from build123d import *

# Parameters (mm, degrees)
SKETCH2_R           = 17.4
SKETCH2_R_2         = 4.45
BOSS_EXTRUDE1_DEPTH = 4


with BuildPart() as part:
    # Sketch2 → Boss-Extrude1 (new body)
    with BuildSketch(Plane.XY):
        Polygon((53.044712849, 33.544372616), (42.778880935, 33.544372616), (42.778880935, 29.544372616), (2.778880935, 29.544372616), (2.778880935, 33.544372616), (-57.221119065, 33.544372616), (-57.221119065, 29.544372616), (-97.221119065, 29.544372616), (-97.221119065, 33.544372616), (-157.221119065, 33.544372616), (-157.221119065, 29.544372616), (-197.221119065, 29.544372616), (-197.221119065, 33.544372616), (-207.486950979, 33.544372616), (-217.221119065, -17.455627384), (-217.221119065, -21.455627384), (-197.221119065, -21.455627384), (-197.221119065, -17.455627384), (-157.221119065, -17.455627384), (-157.221119065, -21.455627384), (-97.221119065, -21.455627384), (-97.221119065, -17.455627384), (-57.221119065, -17.455627384), (-57.221119065, -21.455627384), (2.778880935, -21.455627384), (2.778880935, -17.455627384), (42.778880935, -17.455627384), (42.778880935, -21.455627384), (62.778880935, -21.455627384), (62.778880935, -17.455627384), align=None)
        with Locations((-105.221119065, 4.044372616)):
            Circle(SKETCH2_R, mode=Mode.SUBTRACT)
        with Locations((-130.864831745, -8.505627384)):
            Circle(SKETCH2_R_2, mode=Mode.SUBTRACT)
        with Locations((-79.577406385, 16.594372616)):
            Circle(SKETCH2_R_2, mode=Mode.SUBTRACT)
        with Locations((-74.864831745, -8.505627384)):
            Circle(SKETCH2_R_2, mode=Mode.SUBTRACT)
        with Locations((-49.221119065, 4.044372616)):
            Circle(SKETCH2_R, mode=Mode.SUBTRACT)
        with Locations((-23.577406385, 16.594372616)):
            Circle(SKETCH2_R_2, mode=Mode.SUBTRACT)
        with BuildLine():
            Line((-16.476478057, 4.792165998), (-25.639690827, -7.001469778))
            ThreePointArc((-25.639690827, -7.001469778), (-26.073848783, -11.213946123), (-22.481034397, -13.455627384))
            Line((-22.481034397, -13.455627384), (9.665493618, -13.455627384))
            ThreePointArc((9.665493618, -13.455627384), (13.553631861, -10.39497876), (11.491657622, -5.896817888))
            Line((11.491657622, -5.896817888), (-11.491657622, 5.896817888))
            ThreePointArc((-11.491657622, 5.896817888), (-14.183239425, 6.243267926), (-16.476478057, 4.792165998))
        make_face(mode=Mode.SUBTRACT)
        with BuildLine():
            Line((-165.933895752, 18.177294134), (-142.950580507, 6.383658359))
            ThreePointArc((-142.950580507, 6.383658359), (-140.258998705, 6.03720832), (-137.965760073, 7.488310249))
            Line((-137.965760073, 7.488310249), (-128.802547302, 19.281946025))
            ThreePointArc((-128.802547302, 19.281946025), (-128.368389347, 23.49442237), (-131.961203733, 25.736103631))
            Line((-131.961203733, 25.736103631), (-164.107731748, 25.736103631))
            ThreePointArc((-164.107731748, 25.736103631), (-167.995869991, 22.675455007), (-165.933895752, 18.177294134))
        make_face(mode=Mode.SUBTRACT)
        with BuildLine():
            Line((38.778880935, -4.35874426), (38.778880935, 23.243985793))
            ThreePointArc((38.778880935, 23.243985793), (37.232462018, 26.403090076), (33.788911001, 27.119545047))
            Line((33.788911001, 27.119545047), (-2.125102454, 17.94569653))
            ThreePointArc((-2.125102454, 17.94569653), (-5.110068026, 14.517225335), (-2.961296525, 10.511327779))
            Line((-2.961296525, 10.511327779), (32.952716931, -7.917553756))
            ThreePointArc((32.952716931, -7.917553756), (36.863988125, -7.772294905), (38.778880935, -4.35874426))
        make_face(mode=Mode.SUBTRACT)
        with BuildLine():
            Line((-188.231149131, -14.839068801), (-152.317135675, -5.665220283))
            ThreePointArc((-152.317135675, -5.665220283), (-149.332170104, -2.236749089), (-151.480941605, 1.769148467))
            Line((-151.480941605, 1.769148467), (-187.394955061, 20.198030003))
            ThreePointArc((-187.394955061, 20.198030003), (-191.306226254, 20.052771152), (-193.221119065, 16.639220507))
            Line((-193.221119065, 16.639220507), (-193.221119065, -10.963509547))
            ThreePointArc((-193.221119065, -10.963509547), (-191.674700148, -14.122613829), (-188.231149131, -14.839068801))
        make_face(mode=Mode.SUBTRACT)
    extrude(amount=BOSS_EXTRUDE1_DEPTH)


solid = part.part
Build history of the part. All positions in model axes, mm. A direction names the side the tool comes from. Give positions to 0.01 mm unless a question says otherwise; leave off trailing zeros. Order: outer loops, then holes, each group sorted by start corner. A loop starts at its lowest first (then second) coordinate and runs counter-clockwise, first axis right, second up. Notation, with made-up numbers: M 71.5,79.5 L 81.5,79.5 A22 ccw 81.5,109.5 Z; hole C -13,-21 d1. An arc over 180 degrees is marked long. Put each result on its own line as item: value.
Item 1: Slice it at B-B, the plane x = 28. Write the cut outline in (y, z).
From the geometry:
outline: M -17.46,0 L -5.38,0 L -5.38,4 L -17.46,4 Z; M 25.64,0 L 29.54,0 L 29.54,4 L 25.64,4 Z
Item 2: Probe line 1 (Y direction, x = -138, z = 3.6); line 2 (Y direction, x = -45.5, z = 0.8); line 3 (X direction, y = 2, z = 1.75). List the from-to ranges inside material, lowest first. Write a range as [from, to].
From the geometry:
line 1: y = [-21.46, 7.44], [25.74, 33.54]
line 2: y = [-21.46, -12.95], [21.04, 33.54]
line 3: x = [-213.51, -193.22], [-151.93, -122.5], [-87.94, -66.5], [-31.94, -18.65], [-3.9, 13.63], [38.78, 59.07]
Item 3: Slice it at A-A, the plane x = -49. Write the cut outline in (y, z).
From the geometry:
outline: M -21.46,0 L -13.35,0 L -13.35,4 L -21.46,4 Z; M 21.44,0 L 33.54,0 L 33.54,4 L 21.44,4 Z
Item 4: Two-plate mould, pull along Y, no slides. Class faces 3 (the flat face through (57.98, 7.69, 1.97)), 4 (the flat face through (16.1, 22.6, 2)), 5 (the flat face through (-79, 6, 4)): +Y half, -Y half, draft (parallel to the pull), parting line (faces both ways), or undercut.
From the geometry:
face 3: +Y half
face 4: undercut
face 5: draft
Item 5: Flat gauge pins, fed straight in: pin 1 Ø1 at (y, z) = (-15, 1.5) entering from +X; pin 2 Ø1.2 at (x, z) = (-84, 3) entering from +Y; pin 3 Ø1.2 at (y, z) = (32.5, 2) entering from -X. Where does each tip first touch, or does it go through?
From the geometry:
pin 1: stops at x = 62.41
pin 2: stops at y = 29.54
pin 3: stops at x = -207.8
Item 6: Slice it at C-C, the plane z = 3.2. Give the number of separate pieces and of enclosed holes in the cut face, plus the area to 3 significant figures.
From the geometry:
separate pieces: 1
enclosed holes: 10
area: 8,800 mm2
Item 7: 3-axis set-ups, long thin cutter, end or side, ignore diameter. For faces 1 (the flat face through (-212.286, 8.401, 1.972)), 2 (the flat face through (14.74, 1.43, 1.97)): which of +Z, -Z, +X, -X, +Y, -Y reach the whole face in a straight line?
From the geometry:
face 1: +Z, -Z, -X, +Y
face 2: +Z, -Z
